Work out the finished part from the listing and answer in its coordinate system (mm). Face numbers are marked on the shaded views. A direction names the side the tool comes from. Round coordinates to 2 decimals unless told otherwise and drop trailing zeros. Order: outer loops, then holes, each group sorted by start corner. A loop starts at its lowest first (then second) coordinate and runs counter-clockwise, first axis right, second up. Notation, with made-up numbers: (-6.75, 82.25) - (1.25, 82.25) arc R24 ccw to (1.25, 101.25) - close; hole circle Ø9 at (71, -5.5). An arc over 180 degrees is marked (long way). Use one line per item in the form item = value. Start each with the question number.
Q1. Find the intervals of material crossed by line 1 (Y direction, x = 33.5, z = -6); line 2 (Z direction, x = 4.5, y = -85); line 3 (X direction, y = -41, z = 20.5), in increasing order. Write a range as [from, to].
Q2. The part is cut by section A-A on x = 0. Determine the outline of the cut face in (y, z).
Q3. The part is cut by section C-C on y = -94. Determine the outline of the cut face in (x, z), plus the area to 3 significant figures.
Q4. For a pull along Z with two mould halves and no side action, classify the marked faces 3, 4 and 5 as +Z half, -Z half, draft (parallel to the pull), parting line (faces both ways), or undercut.
Q5. Given P1, Ø2, axis at y = -55, z = -6, coming from the +X side; P2, Ø8, axis at x = -25, z = 18.5, coming from the -Y side; P3, Ø8, axis at y = -120.5, z = 20.5, coming from the +X side, each flat-ended and moving along its own axis, determine where each tip first touches the part or whether it passes through.
Q6. The part is cut by section B-B on y = -118.5. Determine the outline of the cut face in (x, z).
Q7. Which of the six approach directions +Z, -Z, +X, -X, +Y, -Y give full straight-line access (tool end or side, diameter ignored) to the marked faces 1 and 2?
from build123d import *

# Parameters (mm, degrees)
F1_DEPTH  = 31.75
F2_R      = 25.4
F3_DEPTH  = 50.8
F4_SIZE   = 7.62
F5_R      = 18.356615
F3_FACE_R = 17.78
F6_DEPTH  = 101.6


with BuildPart() as f1:
    # F0 (on Front) → F1 (new body)
    with BuildSketch(Plane.XZ):
        Polygon((-18.807561, -32.575652), (18.807561, -32.575652), (37.615123, 0), (18.807561, 32.575652), (-18.807561, 32.575652), (-37.615123, 0), align=None)
    extrude(amount=F1_DEPTH)

    # F2 (on Front) → F3 (join)
    with BuildSketch(Plane.XZ):
        Circle(F2_R)
    extrude(amount=F3_DEPTH)

    # F4
    f4_edges = [f1.edges().sort_by_distance(p)[0] for p in [
        (-25.4, -50.8, 0),
    ]]
    chamfer(f4_edges, length=F4_SIZE)

    # F5 (on Front) + F3_face (on face) → F6 (join)
    with BuildSketch(Plane.XZ):
        Circle(F5_R)
    with BuildSketch(Plane.XZ.offset(50.8)):
        Circle(F3_FACE_R)
    extrude(amount=F6_DEPTH)


solid = f1.part
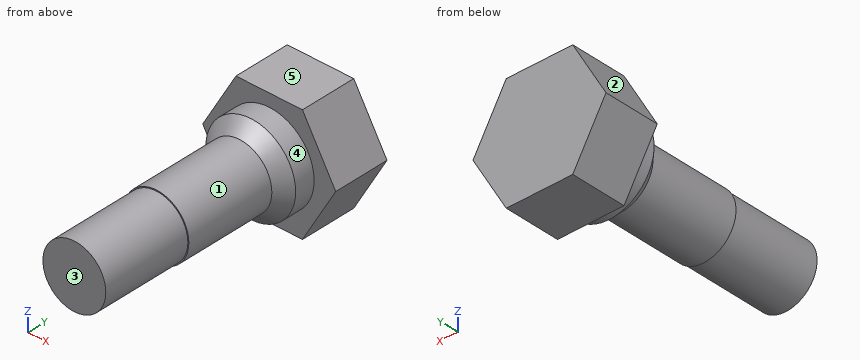
Found:
q1.line_1 = [-31.75, 0]
q1.line_2 = [-17.8, 17.8]
q1.line_3 = [-15, 15]
q2.outline = (-152.4, -17.78) - (-101.6, -17.78) - (-101.6, -18.36) - (-50.22, -18.36) - (-43.18, -25.4) - (-31.75, -25.4) - (-31.75, -32.58) - (0, -32.58) - (0, 32.58) - (-31.75, 32.58) - (-31.75, 25.4) - (-43.18, 25.4) - (-50.22, 18.36) - (-101.6, 18.36) - (-101.6, 17.78) - (-152.4, 17.78) - close
q3.outline = circle Ø36.71 at (0, 0)
q3.area = 1,060 mm²
q4.face_3 = draft
q4.face_4 = parting line
q4.face_5 = +Z half
q5.P1 = 17.66
q5.P2 = -31.75
q5.P3 = 6.62
q6.outline = circle Ø35.56 at (0, 0)
q7.face_1 = -Y
q7.face_2 = +Z, -X, +Y, -Y
